from build123d import *

# Parameters (mm, degrees)
SKETCH1_W           = 22
SKETCH1_H           = 41
BOSS_EXTRUDE1_DEPTH = 101
SKETCH2_R           = 4.1
CUT_EXTRUDE1_DEPTH  = 46


with BuildPart() as part:
    # Sketch1 → Boss-Extrude1 (new, symmetric)
    with BuildSketch(Plane.XY):
        with Locations((0, 20.5)):
            Rectangle(SKETCH1_W, SKETCH1_H)
    extrude(amount=BOSS_EXTRUDE1_DEPTH, both=True)

    # Sketch2 → Cut-Extrude1 (cut, symmetric)
    with BuildSketch(Plane(origin=(0, 0, 0), x_dir=(1, 0, 0), z_dir=(0, 1, 0))):
        with Locations(Location((0, 0, 0), (0, 0, 270))):
            Circle(SKETCH2_R)
    extrude(amount=CUT_EXTRUDE1_DEPTH, both=True, mode=Mode.SUBTRACT)


solid = part.part
Build history of the part. All positions in model axes, mm. Coordinates: 2 decimals unless noted, no trailing zeros. Write each loop counter-clockwise with the first axis right and the second up, starting at its lowest first coordinate (ties: lowest second). Pieces come first, ordered by that corner, then holes.
(1) Cut at A-A on z = 0. List the corners of the cut face in (x, y), and give its area (3 significant figures).
(2) Cut at B-B on x = 0. List the corners of the cut face in (y, z).
(3) Drill centre lines: line 1 (Z direction, x = 0.5, y = 25.5); line 2 (X direction, y = 12.5, z = 0); line 3 (Z direction, x = 1.5, y = 23). Where is each one in solid material? Low to high.
(4) Mould opens along Z. For faces 1 (the cylindrical face through (4.065, 20.787, -0.534)), 2 (the flat face through (0, 21, -101)), 3 (the flat face through (0, 21, 101)) say: pulls with the +Z half, pulls with the -Z half, needs draft (parallel to the pull), parting line crosses it, or undercut.
Working result:
1. outline: (-11, 0) - (-4.1, 0) - (-4.1, 41) - (-11, 41) - close; (4.1, 0) - (11, 0) - (11, 41) - (4.1, 41) - close
1. area: 566 mm2
2. outline: (0, -101) - (41, -101) - (41, -4.1) - (0, -4.1) - close; (0, 4.1) - (41, 4.1) - (41, 101) - (0, 101) - close
3. line 1: z = -101 to -4.07, 4.07 to 101
3. line 2: x = -11 to -4.1, 4.1 to 11
3. line 3: z = -101 to -3.82, 3.82 to 101
4. face 1: undercut
4. face 2: pulls with the -Z half
4. face 3: pulls with the +Z half
